Geometry check sheet. Reference: drawing and pictorial views, mm from the part's lowest x, y, z. A direction names the side the tool comes from. Coordinates: 2 decimals unless noted, no trailing zeros. Write each loop counter-clockwise with the first axis right and the second up, starting at its lowest first coordinate (ties: lowest second). Pieces come first, ordered by that corner, then holes. Notation, with made-up numbers: (22, -28) - (39, -28) arc R32 ccw to (39, 11) - close; hole circle Ø10 at (51.5, 44.25). An arc over 180 degrees is marked (long way). Use one line per item in the form item = value. Start each with the question number.
(1) Tool access check on the marked faces 1 and 2. Record the directions out of +Z, -Z, +X, -X, +Y, -Y that give a thin tool (end or side, any length) a straight path to the whole face; none if there is none.
(2) Sectioned sample at A-A (x = 294). Record the cut outline in (y, z) (3 decimals), and give its area (3 significant figures).
(3) Gauge pin test, flat end, axial feed: pin 1 Ø1 at (y, z) = (156, 15.5) entering from -X. Record the tip position at first contact, or that the pin passes through.
(4) Sectioned sample at C-C (y = 408). Record the cut outline in (x, z) (3 decimals), and give its area (3 significant figures).
(5) Material ranges on line 1 (X direction, y = 136, z = 49.5); line 2 (Y direction, x = 371.5, z = 50); line 3 (Z direction, x = 276.5, y = 294.5) (3 decimals), recorded low to high. Write a range as [from, to].
(6) Sectioned sample at B-B (z = 47). Record the cut outline in (x, y), and give its area (3 significant figures).
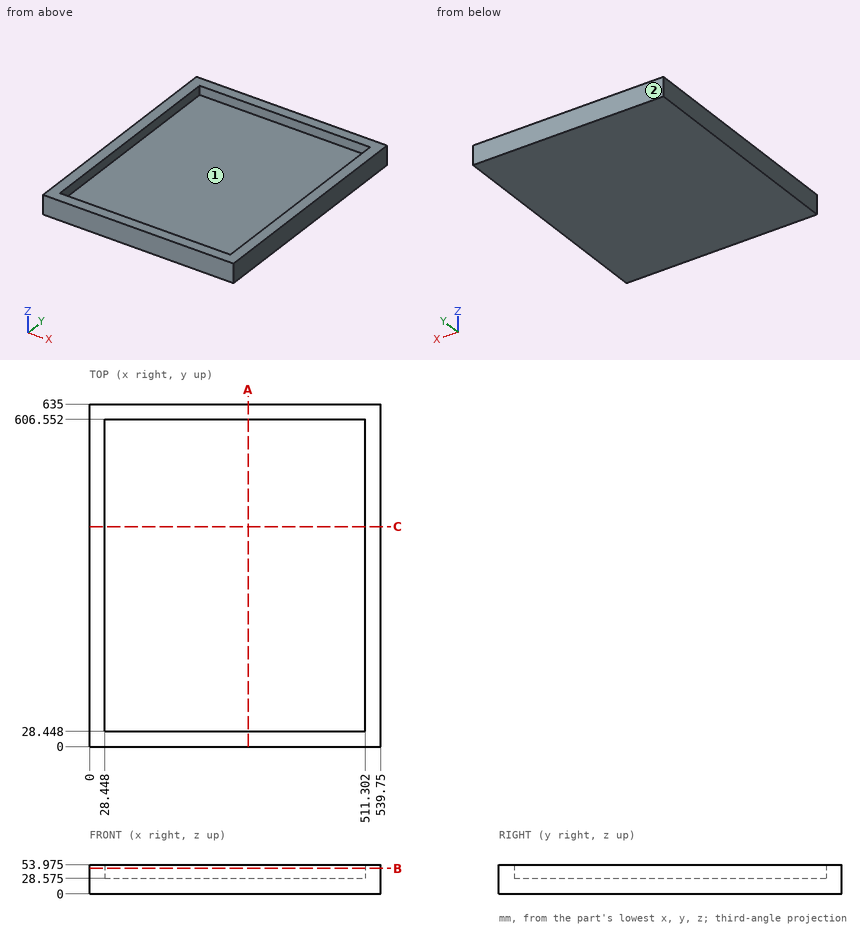
Answers below:
q1.face_1 = +Z
q1.face_2 = +Z, -Z, +X, -X, +Y
q2.outline = (0, 0) - (635, 0) - (635, 53.975) - (606.552, 53.975) - (606.552, 28.575) - (28.448, 28.575) - (28.448, 53.975) - (0, 53.975) - close
q2.area = 19,600 mm2
q3.pin_1 = 0
q4.outline = (0, 0) - (539.75, 0) - (539.75, 53.975) - (511.302, 53.975) - (511.302, 28.575) - (28.448, 28.575) - (28.448, 53.975) - (0, 53.975) - close
q4.area = 16,900 mm2
q5.line_1 = [0, 28.45], [511.3, 539.75]
q5.line_2 = [0, 28.45], [606.55, 635]
q5.line_3 = [0, 28.575]
q6.outline = (0, 0) - (539.75, 0) - (539.75, 635) - (0, 635) - close; hole (28.45, 28.45) - (511.3, 28.45) - (511.3, 606.55) - (28.45, 606.55) - close
q6.area = 63,600 mm2
